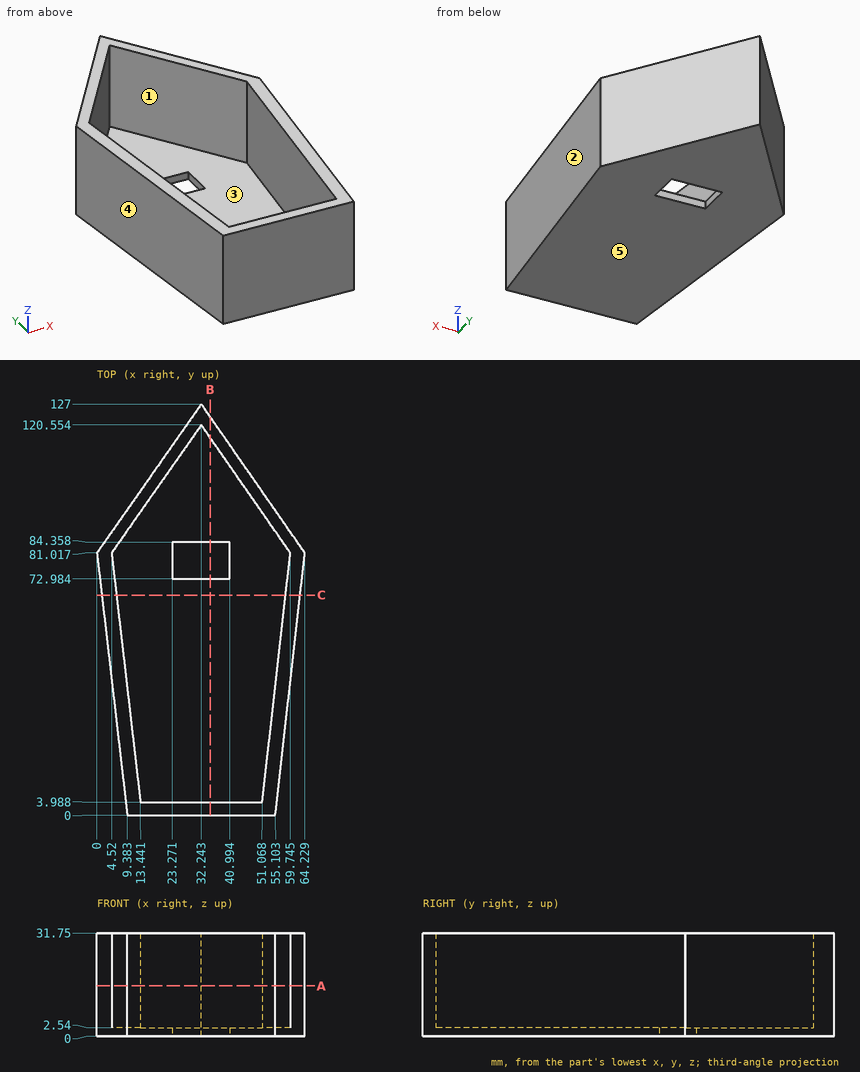
The figure shows three views and two pictorial views of one solid part (mm, origin at its lowest corner). Answer the questions. A direction names the side the tool comes from. Coordinates: 2 decimals unless noted, no trailing zeros. Loops run counter-clockwise (first coordinate to the right, second up) from the corner with the lowest first, then second, coordinate; pieces in that order, holes last. Notation, with made-up numbers: (-21.5, 18.5) -> (21.5, 18.5) arc R28 ccw to (21.5, 36.5) -> close; hole circle Ø11 at (3, 20). An arc over 180 degrees is marked (long way). Use one line per item in the form item = value. Start each with the question number.
Item 1: Consider L1, parallel to Z at x = 13, y = 78; L2, parallel to X at y = 10, z = 30 (1 decimal); L3, parallel to Y at x = 45, z = 11.5 (1 decimal). Determine where each line is inside the solid, lowest interval first. Write a range as [from, to].
Item 2: The mould has two halves that part along Y. Classify the marked faces 3, 4 and 5: released by +Y, released by -Y, zero draft, split by the parting line, or undercut.
Item 3: The part is cut by section B-B on x = 35. Determine the outline of the cut face in (y, z).
Item 4: A tool of negligible diameter and unlimited length cuts with its end or side. For the marked faces 1 and 2, from which of +Z, -Z, +X, -X, +Y, -Y can it reach the whole face along a straight path? Write none if from no direction.
Item 5: Flat-ended cylindrical pins translate along their axes: pin 1 Ø5 at (x, z) = (34, 12) entering from +Y; pin 2 Ø0.8 at (x, z) = (28, 1.5) entering from +Y; pin 3 Ø3 at (y, z) = (77.5, 0.5) entering from +X; pin 4 Ø4 at (x, z) = (42.5, 4) entering from +Y. Find the tip coordinate at first contact, or state that the pin passes through.
Item 6: The part is cut by section A-A on z = 15.5. Determine the outline of the cut face in (x, y) (1 decimal).
Item 7: The part is cut by section C-C on y = 68. Determine the outline of the cut face in (x, z).
Answer key:
q1.L1 = [0, 2.54]
q1.L2 = [8.2, 12.7], [51.7, 56.2]
q1.L3 = [0, 4], [102.2, 108.7]
q2.face_3 = undercut
q2.face_4 = released by -Y
q2.face_5 = zero draft
q3.outline = (0, 0) -> (72.98, 0) -> (72.98, 2.54) -> (3.99, 2.54) -> (3.99, 31.75) -> (0, 31.75) -> close; (84.36, 0) -> (123.04, 0) -> (123.04, 31.75) -> (116.59, 31.75) -> (116.59, 2.54) -> (84.36, 2.54) -> close
q4.face_1 = +Z
q4.face_2 = +Z, -Z, +X, -Y
q5.pin_1 = 127
q5.pin_2 = 121.52
q5.pin_3 = 64
q5.pin_4 = 115.13
q6.outline = (0, 81) -> (9.4, 0) -> (55.1, 0) -> (64.2, 81) -> (32.2, 127) -> close; hole (4.5, 81) -> (13.4, 4) -> (51.1, 4) -> (59.7, 81) -> (32.2, 120.6) -> close
q7.outline = (1.51, 0) -> (62.76, 0) -> (62.76, 31.75) -> (58.28, 31.75) -> (58.28, 2.54) -> (6.03, 2.54) -> (6.03, 31.75) -> (1.51, 31.75) -> close
